```python
from build123d import *

# Parameters (mm, degrees)
SKETCH1_W           = 19.05
SKETCH1_H           = 38.1
SKETCH1_W_2         = 12.7
SKETCH1_H_2         = 31.75
BOSS_EXTRUDE1_DEPTH = 12.7
SKETCH2_R           = 2.54
CUT_EXTRUDE1_DEPTH  = 76.2
SKETCH3_R           = 3.175
CUT_EXTRUDE2_DEPTH  = 30.784140075
SKETCH4_W           = 25.4
SKETCH4_H           = 7.62
CUT_EXTRUDE3_DEPTH  = 30.784140075
SKETCH5_R           = 1.27
CUT_EXTRUDE4_DEPTH  = 35.366350184


with BuildPart() as part:
    # Sketch1 → Boss-Extrude1 (new, symmetric)
    with BuildSketch(Plane.XY):
        Rectangle(SKETCH1_W, SKETCH1_H)
        Rectangle(SKETCH1_W_2, SKETCH1_H_2, mode=Mode.SUBTRACT)
    extrude(amount=BOSS_EXTRUDE1_DEPTH, both=True)

    # Sketch2 → Cut-Extrude1 (cut)
    with BuildSketch(Plane.XZ.offset(19.05)):
        with Locations(Location((0, 0, 0), (0, 0, 270))):
            Circle(SKETCH2_R)
    extrude(amount=-CUT_EXTRUDE1_DEPTH, mode=Mode.SUBTRACT)

    # Sketch3 → Cut-Extrude2 (cut, through all)
    with BuildSketch(Plane(origin=(9.525, 0, 0), x_dir=(0, 0, -1), z_dir=(1, 0, 0))):
        with Locations((-4.7625, -1.27)):
            Circle(SKETCH3_R)
    extrude(amount=-CUT_EXTRUDE2_DEPTH, mode=Mode.SUBTRACT)

    # Sketch4 → Cut-Extrude3 (cut, through all)
    with BuildSketch(Plane(origin=(9.525, 0, 0), x_dir=(0, 0, -1), z_dir=(1, 0, 0))):
        with Locations((0, 15.24)):
            Rectangle(SKETCH4_W, SKETCH4_H)
    extrude(amount=-CUT_EXTRUDE3_DEPTH, mode=Mode.SUBTRACT)

    # Sketch5 → Cut-Extrude4 (cut, through all)
    with BuildSketch(Plane.XZ.offset(19.05)):
        with Locations(Location((0, -6.35, 0), (0, 0, 270))):
            Circle(SKETCH5_R)
        with Locations(Location((0, 6.35, 0), (0, 0, 270))):
            Circle(SKETCH5_R)
    extrude(amount=-CUT_EXTRUDE4_DEPTH, mode=Mode.SUBTRACT)


solid = part.part
```
Design review of the part built by this model. Coordinates are the model's own, in mm. A direction names the side the tool comes from. Coordinates: 2 decimals unless noted, no trailing zeros. Order: outer loops, then holes, each group sorted by start corner. A loop starts at its lowest first (then second) coordinate and runs counter-clockwise, first axis right, second up. Notation, with made-up numbers: M 10,58 L 20,58 A13 ccw 20,69 Z; hole C 33.25,42.25 d6. An arc over 180 degrees is marked long. Answer as a JSON object with one key per item and string values. Group by question number.
1) Wall thickness on L1, parallel to X at y = 2.5, z = -7.5 (3 decimals); L2, parallel to X at y = -18, z = 6.35 (3 decimals); L3, parallel to Y at x = -2.5, z = 8.75 (3 decimals): over which ranges is each line inside the solid? List them lowest first.
2) Add section C-C, the plane x = 0. Write out the cut boundary in (y, z) (3 decimals), then the cut area to 3 significant figures.
3) Tool access review of faces 4 (the flat face through (3, -15.875, 0)), 5 (the flat face through (8, 11.43, 0)): name each direction out of +Z, -Z, +X, -X, +Y, -Y from which nothing blocks a thin tool from reaching the whole face with its end or side.
4) Add section D-D, the plane y = 9.5. Write out the cut boundary in (x, z) (3 decimals), then the cut area to 3 significant figures.
5) Add section B-B, the plane z = 0. Write out the cut boundary in (x, y) (3 decimals), then the cut area to 3 significant figures.
6) Add section A-A, the plane y = -1.27. Count the separate pieces of the cut face and the enclosed holes in it, then the cut area to 3 significant figures.
7) For pin 1 (4 mm diameter, centred on x = 0, z = 0, fed in from -Y); pin 2 (3 mm diameter, centred on x = 0, z = 6.35, fed in from +Y) (3 decimals), all flat-tipped, find the tip position at first contact; note any pin that passes through.
8) Mouldability with a two-part tool opening along Z and no side actions: class faces 1 (the flat face through (-6.35, -2, 0)), 2 (the cylindrical face through (-7.915, -0.316, 1.734)), 3 (the flat face through (-6.5, -7, -12.7)) as pulls with the +Z half, pulls with the -Z half, needs draft (parallel to the pull), parting line crosses it, or undercut.
Computed values:
{
 "1": {"L1": "x = -9.525 to -6.35, 6.35 to 9.525", "L2": "x = -9.525 to -1.27, 1.27 to 9.525", "L3": "y = -19.05 to -15.875"},
 "2": {"outline": "M -19.05,-12.7 L -15.875,-12.7 L -15.875,-7.62 L -19.05,-7.62 Z; M -19.05,-5.08 L -15.875,-5.08 L -15.875,-2.54 L -19.05,-2.54 Z; M -19.05,2.54 L -15.875,2.54 L -15.875,5.08 L -19.05,5.08 Z; M -19.05,7.62 L -15.875,7.62 L -15.875,12.7 L -19.05,12.7 Z", "area": "48.4 mm^2"},
 "3": {"face 4": "+Z, -Z, +Y", "face 5": "+Z, -Z, +X, -X, +Y"},
 "4": {"outline": "M -9.525,-12.7 L -6.35,-12.7 L -6.35,12.7 L -9.525,12.7 Z; M 6.35,-12.7 L 9.525,-12.7 L 9.525,12.7 L 6.35,12.7 Z", "area": "161 mm^2"},
 "5": {"outline": "M -9.525,-19.05 L -2.54,-19.05 L -2.54,-15.875 L -6.35,-15.875 L -6.35,11.43 L -9.525,11.43 Z; M 2.54,-19.05 L 9.525,-19.05 L 9.525,11.43 L 6.35,11.43 L 6.35,-15.875 L 2.54,-15.875 Z", "area": "218 mm^2"},
 "6": {"separate pieces": "4", "enclosed holes": "0", "area": "121 mm^2"},
 "7": {"pin 1": "passes through", "pin 2": "stops at y = -15.875"},
 "8": {"face 1": "needs draft", "face 2": "undercut", "face 3": "pulls with the -Z half"}
}
